```python
from build123d import *

# Parameters (mm, degrees)
F0_R     = 6.0866726669
F1_DEPTH = 2032
F2_W     = 12.4690905213
F2_H     = 123.6518211663
F3_DEPTH = 5.334
F4_W     = 14.5472697914
F4_H     = 136.9002275169
F5_DEPTH = 6.096
F6_W     = 6.096
F6_H     = 14.5472697914
F7_DEPTH = 762
F8_W     = 5.334
F8_H     = 12.4690905213
F9_DEPTH = 762


with BuildPart() as f1:
    # F0 (on Right) → F1 (new body)
    with BuildSketch(Plane.YZ):
        with Locations((-52.2143170238, 53.5131841898)):
            Circle(F0_R)
    extrude(amount=F1_DEPTH)

    # F2 (on Right) → F3 (join)
    with BuildSketch(Plane.YZ):
        with Locations((-52.214320749, -4.156364128)):
            Rectangle(F2_W, F2_H)
    extrude(amount=F3_DEPTH)

    # F4 (on face) → F5 (join)
    with BuildSketch(Plane.YZ.offset(2032)):
        with Locations((-52.2143188864, -10.5207953602)):
            Rectangle(F4_W, F4_H)
    extrude(amount=F5_DEPTH)

    # F6 (on face) → F7 (join)
    with BuildSketch(Plane(origin=(0, 0, -78.9709091187), x_dir=(1, 0, 0), z_dir=(0, 0, -1))):
        with Locations((2035.048, 52.2143188864)):
            Rectangle(F6_W, F6_H)
    extrude(amount=F7_DEPTH)

    # F8 (on face) → F9 (join)
    with BuildSketch(Plane(origin=(0, 0, -65.9822747111), x_dir=(1, 0, 0), z_dir=(0, 0, -1))):
        with Locations((2.667, 52.214320749)):
            Rectangle(F8_W, F8_H)
    extrude(amount=F9_DEPTH)


solid = f1.part
```
Can you work these out from the model? Positions are in its coordinate system, mm. Round coordinates to 2 decimals unless told otherwise and drop trailing zeros. Loops run counter-clockwise (first coordinate to the right, second up) from the corner with the lowest first, then second, coordinate; pieces in that order, holes last. Notation, with made-up numbers: (1, 58.5) -> (46, 58.5) arc R16 ccw to (46, 66.5) -> close; hole circle Ø9 at (28.5, -3). An arc over 180 degrees is marked (long way). One line per item, written item: value. Start each with the question number.
1. If we section it at C-C, the plane x = 186.5: Write out the boundary of the cut face in (y, z).
2. For pin 1 (1.5 mm diameter, centred on x = 280, y = -51.5, fed in from -Z); pin 2 (1.6 mm diameter, centred on x = 3, y = -51, fed in from -Z); pin 3 (1.5 mm diameter, centred on x = 372.5, y = -56.5, fed in from +Z), each with a flat end and sliding along its axis, tell me the tip position at first contact or that it passes through.
3. If we section it at A-A, the plane z = -314: Write out the boundary of the cut face in (x, y), then the cut area to 3 significant figures.
4. If we section it at B-B, the plane y = -51: Write out the boundary of the cut face in (x, z), then the cut area to 3 significant figures.
5. If I drill on probe 1 along X at (y, z) = (-57, -290); probe 2 along Z at (x, y) = (395.5, -53.5); probe 3 along Z at (x, y) = (820.5, -54), over which ranges is the centre line in solid material (lowest first)?
Calculated:
1. outline: circle Ø12.17 at (-52.21, 53.51)
2. pin 1: stops at z = 47.43
2. pin 2: stops at z = -827.98
2. pin 3: stops at z = 58.47
3. outline: (0, -58.45) -> (5.33, -58.45) -> (5.33, -45.98) -> (0, -45.98) -> close; (2032, -59.49) -> (2038.1, -59.49) -> (2038.1, -44.94) -> (2032, -44.94) -> close
3. area: 155 mm²
4. outline: (0, -827.98) -> (5.33, -827.98) -> (5.33, 47.55) -> (2032, 47.55) -> (2032, -840.97) -> (2038.1, -840.97) -> (2038.1, 57.93) -> (2032, 57.93) -> (2032, 59.48) -> (0, 59.48) -> close
4. area: 34,400 mm²
5. probe 1: x = 0 to 5.33, 2032 to 2038.1
5. probe 2: z = 47.56 to 59.46
5. probe 3: z = 47.69 to 59.33
